Check sheet for the modelled part. Datum: model origin and axes. Units: mm. Face numbers are marked on the shaded views. A direction names the side the tool comes from. Round coordinates to 2 decimals unless told otherwise and drop trailing zeros. Write each loop counter-clockwise with the first axis right and the second up, starting at its lowest first coordinate (ties: lowest second). Pieces come first, ordered by that corner, then holes. Notation, with made-up numbers: M -9,66 L 37,66 A27 cw 37,98 Z; hole C 5,-2.75 d1. An arc over 180 degrees is marked long. Put each result on its own line as item: value.
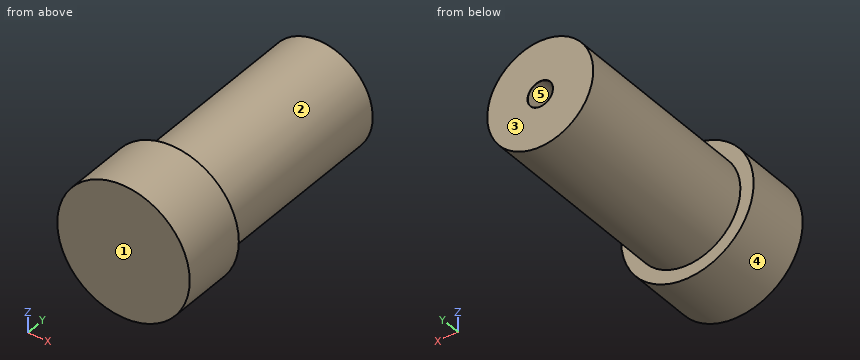
```python
from build123d import *

# Parameters (mm, degrees)
SKETCH1_R                            = 10
BOSS_EXTRUDE1_DEPTH                  = 40
F_3_8_3_8_DIAMETER_HOLE1_D           = 3.8
F_3_8_3_8_DIAMETER_HOLE1_DEPTH       = 15
F_3_8_3_8_DIAMETER_HOLE1_CSINK_D     = 3.85
F_3_8_3_8_DIAMETER_HOLE1_CSINK_ANGLE = 90
F_3_8_3_8_DIAMETER_HOLE1_TIP         = 1.141635176
SKETCH5_R                            = 13.85296062
SKETCH5_R_2                          = 8
CUT_EXTRUDE1_DEPTH                   = 30


with BuildPart() as part:
    # Sketch1 → Boss-Extrude1 (new body)
    with BuildSketch(Plane(origin=(0, 0, 0), x_dir=(1, 0, 0), z_dir=(0, 1, 0))):
        with Locations(Location((0, 0, 0), (0, 0, 270))):
            Circle(SKETCH1_R)
    extrude(amount=BOSS_EXTRUDE1_DEPTH)

    # Ø3.8 (3.8) Diameter Hole1
    with Locations(Plane(origin=(0, 40, 0), x_dir=(1, 0, 0), z_dir=(0, 1, 0))):
        with Locations((0, 0)):
            CounterSinkHole(F_3_8_3_8_DIAMETER_HOLE1_D / 2, F_3_8_3_8_DIAMETER_HOLE1_CSINK_D / 2, depth=F_3_8_3_8_DIAMETER_HOLE1_DEPTH, counter_sink_angle=F_3_8_3_8_DIAMETER_HOLE1_CSINK_ANGLE)
            with Locations((0, 0, -(F_3_8_3_8_DIAMETER_HOLE1_DEPTH + F_3_8_3_8_DIAMETER_HOLE1_TIP / 2))):  # 118° drill point
                Cone(0, F_3_8_3_8_DIAMETER_HOLE1_D / 2, F_3_8_3_8_DIAMETER_HOLE1_TIP, mode=Mode.SUBTRACT)

    # Sketch5 → Cut-Extrude1 (cut)
    with BuildSketch(Plane(origin=(0, 40, 0), x_dir=(1, 0, 0), z_dir=(0, 1, 0))):
        Circle(SKETCH5_R)
        with Locations(Location((0, 0, 0), (0, 0, 270))):
            Circle(SKETCH5_R_2, mode=Mode.SUBTRACT)
    extrude(amount=-CUT_EXTRUDE1_DEPTH, mode=Mode.SUBTRACT)


solid = part.part
```
1. Cross-section at A-A (z = -6.25). Enter the section's corners in (x, y).
Computed values:
outline: M -7.81,0 L 7.81,0 L 7.81,10 L 4.99,10 L 4.99,40 L -4.99,40 L -4.99,10 L -7.81,10 Z
2. Depth check by flat-ended pin: pin 1 Ø8 at (x, y) = (7, 32) entering from +Z; pin 2 Ø2 at (x, y) = (3.5, 5.5) entering from +Z; pin 3 Ø5 at (x, y) = (-6, 16.5) entering from -Z. Enter the tip coordinate at first touch or a pass-through.
Computed values:
pin 1: stops at z = 7.42
pin 2: stops at z = 9.68
pin 3: stops at z = -7.19
3. Scan lines: probe 1 along Y at (x, z) = (-8.25, -4.5); probe 2 along Z at (x, y) = (-6, 7); probe 3 along Z at (x, y) = (0.25, 3.5). Record each from-to range of solid material in increasing order.
Computed values:
probe 1: y = 0 to 10
probe 2: z = -8 to 8
probe 3: z = -10 to 10
4. Release check for a two-part mould opening along X. For the marked faces 3, 4 and 5 record: +X half, -X half, draft (parallel to the pull), parting line (faces both ways), or undercut.
Computed values:
face 3: draft
face 4: parting line
face 5: undercut
5. Cross-section at B-B (x = 7). Enter the section's corners in (y, z), then the cut area to 3 significant figures.
Computed values:
outline: M 0,-7.14 L 10,-7.14 L 10,-3.87 L 40,-3.87 L 40,3.87 L 10,3.87 L 10,7.14 L 0,7.14 Z
area: 375 mm2
6. Access from +Z, -Z, +X, -X, +Y, -Y to the whole of each face (thin tool, end or side, straight path). Record for the marked faces 1 and 2.
Computed values:
face 1: +Z, -Z, +X, -X, -Y
face 2: +Y
7. Cross-section at C-C (y = 13.5). Enter the section's corners in (x, z), then the cut area to 3 significant figures.
Computed values:
outline: C 0,0 d16
area: 201 mm2
8. Cross-section at D-D (z = 8.5). Enter the section's corners in (x, y), then the cut area to 3 significant figures.
Computed values:
outline: M -5.27,0 L 5.27,0 L 5.27,10 L -5.27,10 Z
area: 105 mm2
